CAD build for the part. Positions are in the model's coordinates, mm. A direction names the side the tool comes from. Coordinates: 2 decimals unless noted, no trailing zeros. Write each loop counter-clockwise with the first axis right and the second up, starting at its lowest first coordinate (ties: lowest second). Pieces come first, ordered by that corner, then holes.
```python
from build123d import *

# Parameters (mm, degrees)
F0_R      = 16.5
F0_R_2    = 15
F1_DEPTH  = 3
F2_R      = 16.5
F2_R_2    = 15
F3_DEPTH  = 62
F4_R      = 3.5
F5_DEPTH  = 62
F7_W      = 7
F7_H      = 31
F8_DEPTH  = 20
F11_DEPTH = 1.5
F12_R     = 2


with BuildPart() as f1:
    # F0 (on Top) → F1 (new body)
    with BuildSketch(Plane.XY):
        Circle(F0_R)
        Circle(F0_R_2, mode=Mode.SUBTRACT)
        Circle(F0_R_2)
    extrude(amount=F1_DEPTH)

    # F2 (on face) → F3 (join)
    with BuildSketch(Plane.XY.offset(3)):
        Circle(F2_R)
        Circle(F2_R_2, mode=Mode.SUBTRACT)
    extrude(amount=F3_DEPTH)

    # F4 (on face) → F5 (join)
    with BuildSketch(Plane.XY.offset(3)):
        Circle(F4_R)
    extrude(amount=F5_DEPTH)

    # F7 (on offset) → F8 (cut)
    with BuildSketch(Plane.XZ.offset(30)):
        with Locations((0, 31)):
            Rectangle(F7_W, F7_H)
    extrude(amount=-F8_DEPTH, mode=Mode.SUBTRACT)

    # F10 (on offset) → F11 (join, symmetric)
    with BuildSketch(Plane.XZ.offset(16.5)):
        with BuildLine():
            Line((0.5, 65), (0, 65))
            Line((0, 65), (-0.5, 65))
            ThreePointArc((-0.5, 65), (-0.853553, 64.853553), (-1, 64.5))
            Line((-1, 64.5), (-1, 62))
            ThreePointArc((-1, 62), (-0.853553, 61.646447), (-0.5, 61.5))
            Line((-0.5, 61.5), (0.5, 61.5))
            ThreePointArc((0.5, 61.5), (0.853553, 61.646447), (1, 62))
            Line((1, 62), (1, 64.5))
            ThreePointArc((1, 64.5), (0.853553, 64.853553), (0.5, 65))
        make_face()
    extrude(amount=F11_DEPTH, both=True)

    # F12
    f12_edges = [f1.edges().sort_by_distance(p)[0] for p in [
        (-16.5, 0, 0),
    ]]
    fillet(f12_edges, radius=F12_R)


solid = f1.part
```
Item 1: Which spindle directions (+Z, -Z, +X, -X, +Y, -Y) get a long thin tool onto all of the face, cutting with end or side? Do faces 4 (the cylindrical face through (3.233, -1.341, 33.566)), 5 (the flat face through (1, -17, 63)), 6 (the flat face through (0, -16, 15.5)). Say none if no direction does.
Item 2: Wall check: line 1 along X through (y, z) = (1.5, 45); line 2 along Y through (x, z) = (0, 19); line 3 along X through (y, z) = (2, 53.5). Give the ranges that are in metal, low to high.
Item 3: Saw through at B-B, the plane y = 0. Write the cut outline in (x, z), and give its area (3 significant figures).
Item 4: Two-plate mould, pull along Y, no slides. Class faces 1 (the flat face through (0, 0, 65)), 2 (the flat face through (0, 4, 3)), 3 (the cylindrical face through (15.24, -6.32, 33.06)): +Y half, -Y half, draft (parallel to the pull), parting line (faces both ways), or undercut.
Item 5: Saw through at A-A, the plane z = 38. Write the cut outline in (x, y).
Item 6: Flat gauge pins, fed straight in: pin 1 Ø1.2 at (y, z) = (-15.5, 25) entering from +X; pin 2 Ø1.5 at (x, z) = (1.5, 50.5) entering from -Y; pin 3 Ø5 at (y, z) = (-8, 15) entering from +X. Where does each tip first touch, or does it go through?
Working result:
1. face 4: +Z
1. face 5: +Z, -Z, +X, -Y
1. face 6: -Y
2. line 1: x = -16.43 to -14.92, -3.16 to 3.16, 14.92 to 16.43
2. line 2: y = -3.5 to 3.5, 15 to 16.5
2. line 3: x = -16.38 to -14.87, -2.87 to 2.87, 14.87 to 16.38
3. outline: (-16.5, 2) arc R2 ccw to (-14.5, 0) - (14.5, 0) arc R2 ccw to (16.5, 2) - (16.5, 65) - (15, 65) - (15, 3) - (3.5, 3) - (3.5, 65) - (-3.5, 65) - (-3.5, 3) - (-15, 3) - (-15, 65) - (-16.5, 65) - close
3. area: 717 mm2
4. face 1: draft
4. face 2: undercut
4. face 3: parting line
5. outline: (-3.5, -16.12) - (-3.5, -14.59) arc R15 cw (long way) to (3.5, -14.59) - (3.5, -16.12) arc R16.5 ccw (long way) to start; circle Ø7 at (0, 0)
6. pin 1: stops at x = 7.09
6. pin 2: stops at y = -16.48
6. pin 3: stops at x = 15.56
